```python
from build123d import *

# Parameters (mm, degrees)
SKETCH1_W               = 76.2
SKETCH1_H               = 69.85
BOSS_EXTRUDE1_DEPTH     = 9.525
F_1_4_CLEARANCE_HOLE1_D = 6.7564
SKETCH5_W               = 11.2395
SKETCH5_H               = 11.2395
CUT_EXTRUDE1_DEPTH      = 6.8326
F_3_8_CLEARANCE_HOLE1_D = 13.97
CUT_EXTRUDE2_START      = -6.35
CUT_EXTRUDE2_DEPTH      = 6.8326
MIRROR2_START           = -6.35
MIRROR2_COPY_2_DEPTH    = 6.8326


with BuildPart() as part:
    # Sketch1 → Boss-Extrude1 (new, symmetric)
    with BuildSketch(Plane(origin=(0, 0, 0), x_dir=(1, 0, 0), z_dir=(0, 1, 0))):
        Rectangle(SKETCH1_W, SKETCH1_H)
    extrude(amount=BOSS_EXTRUDE1_DEPTH, both=True)

    # 1/4 Clearance Hole1 (through all)
    with Locations(Plane(origin=(0, 9.525, 0), x_dir=(1, 0, 0), z_dir=(0, 1, 0))):
        with Locations((-15.875, 15.875)):
            f_1_4_clearance_hole1 = Hole(F_1_4_CLEARANCE_HOLE1_D / 2)

    # Sketch5 → Cut-Extrude1 (cut)
    with BuildSketch(Plane(origin=(0, 9.525, 0), x_dir=(1, 0, 0), z_dir=(0, 1, 0))):
        with Locations((-15.875, 15.875)):
            Rectangle(SKETCH5_W, SKETCH5_H)
    cut_extrude1 = extrude(amount=-CUT_EXTRUDE1_DEPTH, mode=Mode.SUBTRACT)

    # Sketch-Pattern1: 1/4 Clearance Hole1, Cut-Extrude1 at 3 more places
    with Locations((31.75, 0, 0), (31.75, 0, 31.75), (0, 0, 31.75)):
        add(f_1_4_clearance_hole1, mode=Mode.SUBTRACT)
        add(cut_extrude1, mode=Mode.SUBTRACT)

    # 3/8 Clearance Hole1 (through all)
    with Locations(Plane(origin=(0, 9.525, 0), x_dir=(1, 0, 0), z_dir=(0, 1, 0))):
        with Locations((0, 0)):
            Hole(F_3_8_CLEARANCE_HOLE1_D / 2)


with BuildPart() as body_2:
    # uxcell-FR6ZZ: read off the stored shape, not the designer's step
    # uxcell-FR6ZZ outline → uxcell-FR6ZZ (revolve)
    with BuildSketch(Plane(origin=(-26.978230937, 0, 2.629647059), x_dir=(1, 0, 0), z_dir=(0, 0, 1))):
        Polygon((12.430125, 16.66875), (4.7625, 16.66875), (4.7625, 8.255), (11.2395, 8.255), (11.2395, 13.414375), (11.636375, 13.81125), (12.430125, 13.81125), align=None)
    revolve(axis=Axis((-26.978230937, 0, 2.629647059), (0, 1, 0)))


with BuildPart() as body_2_1:
    # Body-Move/Copy2: read off the stored shape, not the designer's step
    # Body-Move/Copy2: moved
    add(body_2.part.moved(Location((26.9782309, -7.14375, -2.6296471))))


with BuildPart() as part_1:
    add(part.part)

    # Combine1: cut body 2
    add(body_2_1.part, mode=Mode.SUBTRACT)

    # Sketch11 → 1/4 Clearance Hole2 (revolve, cut)
    with BuildSketch(Plane(origin=(-28.575, 0, 34.925), x_dir=(0, -1, 0), z_dir=(1, 0, 0))):
        Polygon((0, 0), (0, 27.429827343), (3.3782, 25.4), (3.3782, 0), align=None)
    f_1_4_clearance_hole2 = revolve(axis=Axis((-28.575, 0, 41.275), (0, 0, -1)), mode=Mode.SUBTRACT)

    # Sketch13 → Cut-Extrude2 (cut)
    with BuildSketch(Plane.XY.offset(34.925).offset(CUT_EXTRUDE2_START)):
        Polygon((-34.19475, 5.61975), (-34.19475, 9.525), (-22.95525, 9.525), (-22.95525, 5.61975), (-22.95525, -5.61975), (-34.19475, -5.61975), align=None)
    cut_extrude2 = extrude(amount=-CUT_EXTRUDE2_DEPTH, mode=Mode.SUBTRACT)

    # Mirror1: 1/4 Clearance Hole2, Cut-Extrude2 across plane
    add(f_1_4_clearance_hole2.mirror(Plane(origin=(0, 0, 0), x_dir=(0, 0, 1), z_dir=(1, 0, 0))), mode=Mode.SUBTRACT)
    add(cut_extrude2.mirror(Plane(origin=(0, 0, 0), x_dir=(0, 0, 1), z_dir=(1, 0, 0))), mode=Mode.SUBTRACT)

    # Mirror2: 1/4 Clearance Hole2, Cut-Extrude2 across plane
    add(f_1_4_clearance_hole2.mirror(Plane.XY), mode=Mode.SUBTRACT)
    add(cut_extrude2.mirror(Plane.XY), mode=Mode.SUBTRACT)

    # Mirror2 copy 1 sketch → Mirror2 copy 1 (revolve, cut)
    with BuildSketch(Plane(origin=(28.575, 0, -34.925), x_dir=(0, -1, 0), z_dir=(-1, 0, 0))):
        Polygon((0, 0), (0, 27.429827343), (3.3782, 25.4), (3.3782, 0), align=None)
    revolve(axis=Axis((28.575, 0, -41.275), (0, 0, 1)), mode=Mode.SUBTRACT)

    # Mirror2 copy 2 sketch → Mirror2 copy 2 (cut)
    with BuildSketch(Plane(origin=(0, 0, -34.925), x_dir=(-1, 0, 0), z_dir=(0, 0, -1)).offset(MIRROR2_START)):
        Polygon((-34.19475, 5.61975), (-34.19475, 9.525), (-22.95525, 9.525), (-22.95525, 5.61975), (-22.95525, -5.61975), (-34.19475, -5.61975), align=None)
    extrude(amount=-MIRROR2_COPY_2_DEPTH, mode=Mode.SUBTRACT)


solid = part_1.part
```
Here's how the part is built. I have some questions about the finished solid (model axes, mm). A direction names the side the tool comes from. Coordinates: 2 decimals unless noted, no trailing zeros. Write each loop counter-clockwise with the first axis right and the second up, starting at its lowest first coordinate (ties: lowest second). Pieces come first, ordered by that corner, then holes. Notation, with made-up numbers: (80, 36.5) -> (121, 36.5) arc R16 ccw to (121, 59.5) -> close; hole circle Ø11 at (60, -24.5). An arc over 180 degrees is marked (long way). Use a Markdown table: item, result. Add a question column.
(1) If we section it at D-D, the plane x = -16: Write out the boundary of the cut face in (y, z) (3 decimals), and give its area (3 significant figures).
(2) For faces 1 (the cylindrical face through (-31.924, 0.44, -31.794)), 2 (the flat face through (28, -5.62, -25)), 3 (the cylindrical face through (-31.924, 0.44, 15.719)), which set-ups out of +Z, -Z, +X, -X, +Y, -Y let a thin tool reach every point of the face, with its end or its side?
(3) Please list where these lines run through material, in increasing order: line 1 (X direction, y = 0, z = -33.5); line 2 (X direction, y = 3.5, z = 15); line 3 (Z direction, x = -29.5, y = 6.5) (3 decimals).
(4) If we section it at A-A, the plane z = 0: Write out the boundary of the cut face in (x, y) (1 decimal).
(5) We'd pull the mould along Y, two halves only. Please class faces 4 (the flat face through (16, 6, -10.255)), 5 (the flat face through (-13, 2.692, 18)), 6 (the cylindrical face through (31.924, 0.44, 15.719)): +Y half, -Y half, draft (parallel to the pull), parting line (faces both ways), or undercut.
(6) If we section it at C-C, the plane z = -25: Write out the boundary of the cut face in (x, y) (3 decimals), and give its area (3 significant figures).
(7) If we section it at B-B, the plane x = 0: Write out the boundary of the cut face in (y, z) (1 decimal).
(8) I'm going to push flat-ended pins straight in: P1, Ø2, axis at x = -30.5, z = 26.5, coming from the +Y side; P2, Ø11, axis at x = 28.575, y = 0, coming from the +Z side (3 decimals); P3, Ø5.5, axis at x = 17, z = 18, coming from the +Y side. Where does each tip first touch, or does it pass through?
Outcome:
| question | item | result |
|---|---|---|
| 1 | outline | (-9.525, -34.925) -> (9.525, -34.925) -> (9.525, -21.495) -> (2.692, -21.495) -> (2.692, -19.251) -> (-9.525, -19.251) -> close; (-9.525, -12.499) -> (2.692, -12.499) -> (2.692, -10.255) -> (9.525, -10.255) -> (9.525, 10.255) -> (2.692, 10.255) -> (2.692, 12.499) -> (-9.525, 12.499) -> close; (-9.525, 19.251) -> (2.692, 19.251) -> (2.692, 21.495) -> (9.525, 21.495) -> (9.525, 34.925) -> (-9.525, 34.925) -> close |
| 1 | area | 1,010 mm^2 |
| 2 | face 1 | -Z |
| 2 | face 2 | +Y |
| 2 | face 3 | +Z |
| 3 | line 1 | x = -38.1 to -31.95, -25.2 to 25.2, 31.95 to 38.1 |
| 3 | line 2 | x = -38.1 to -21.49, -10.26 to 10.26, 21.49 to 38.1 |
| 3 | line 3 | z = -34.925 to -28.575, -21.742 to 21.742, 28.575 to 34.925 |
| 4 | outline | (-38.1, -9.5) -> (-7, -9.5) -> (-7, 1.1) -> (-11.2, 1.1) -> (-11.2, 6.3) -> (-11.6, 6.7) -> (-12.4, 6.7) -> (-12.4, 9.5) -> (-38.1, 9.5) -> close; (7, -9.5) -> (38.1, -9.5) -> (38.1, 9.5) -> (12.4, 9.5) -> (12.4, 6.7) -> (11.6, 6.7) -> (11.2, 6.3) -> (11.2, 1.1) -> (7, 1.1) -> close |
| 5 | face 4 | draft |
| 5 | face 5 | +Y half |
| 5 | face 6 | undercut |
| 6 | outline | (-38.1, -9.525) -> (38.1, -9.525) -> (38.1, 9.525) -> (34.195, 9.525) -> (34.195, -5.62) -> (22.955, -5.62) -> (22.955, 9.525) -> (-22.955, 9.525) -> (-22.955, -5.62) -> (-34.195, -5.62) -> (-34.195, 9.525) -> (-38.1, 9.525) -> close |
| 6 | area | 1,110 mm^2 |
| 7 | outline | (-9.5, -34.9) -> (9.5, -34.9) -> (9.5, -12.4) -> (6.7, -12.4) -> (6.7, -11.6) -> (6.3, -11.2) -> (1.1, -11.2) -> (1.1, -7) -> (-9.5, -7) -> close; (-9.5, 7) -> (1.1, 7) -> (1.1, 11.2) -> (6.3, 11.2) -> (6.7, 11.6) -> (6.7, 12.4) -> (9.5, 12.4) -> (9.5, 34.9) -> (-9.5, 34.9) -> close |
| 8 | P1 | stops at y = -5.62 |
| 8 | P2 | stops at z = 34.925 |
| 8 | P3 | stops at y = 2.69 |
